Design review of the part shown in the three views and the two pictorial views. Dimensions are in mm from the part's minimum x, y and z. Round coordinates to 2 decimals unless told otherwise and drop trailing zeros. Write each loop counter-clockwise with the first axis right and the second up, starting at its lowest first coordinate (ties: lowest second). Pieces come first, ordered by that corner, then holes. Notation, with made-up numbers: (-1, -15.5) - (35, -15.5) arc R10 ccw to (35, 1.5) - close; hole circle Ø7 at (-36.5, 19.5). An arc over 180 degrees is marked (long way). One line per item, written item: value. Start each with the question number.
Q1. Add section C-C on x = 1.5. Write out the cut boundary in (y, z), and give its area (3 significant figures).
Q2. Add section B-B on z = 0.75. Write out the cut boundary in (x, y), and give its area (3 significant figures).
Q3. Clearance check with flat-ended pins moving along their axes: pin 1 Ø3 at (x, y) = (5, 40) entering from +Z; pin 2 Ø1.5 at (x, z) = (1, 3) entering from -Y. State where each tip first meets the part, or that it passes through.
Q4. For probe 1 along Y at (x, z) = (5.5, 2.9); probe 2 along Y at (x, z) = (3.25, 4.2); probe 3 along X at (y, z) = (4, 3.8), list the stretches that pass through material, from the lowest coordinate up.
Q5. Add section A-A on x = 5. Write out the cut boundary in (y, z), and give its area (3 significant figures).
Q6. Mouldability with a two-part tool opening along Y and no side actions: class the marked faces 1, 2 and 3 as +Y half, -Y half, draft (parallel to the pull), parting line (faces both ways), or undercut.
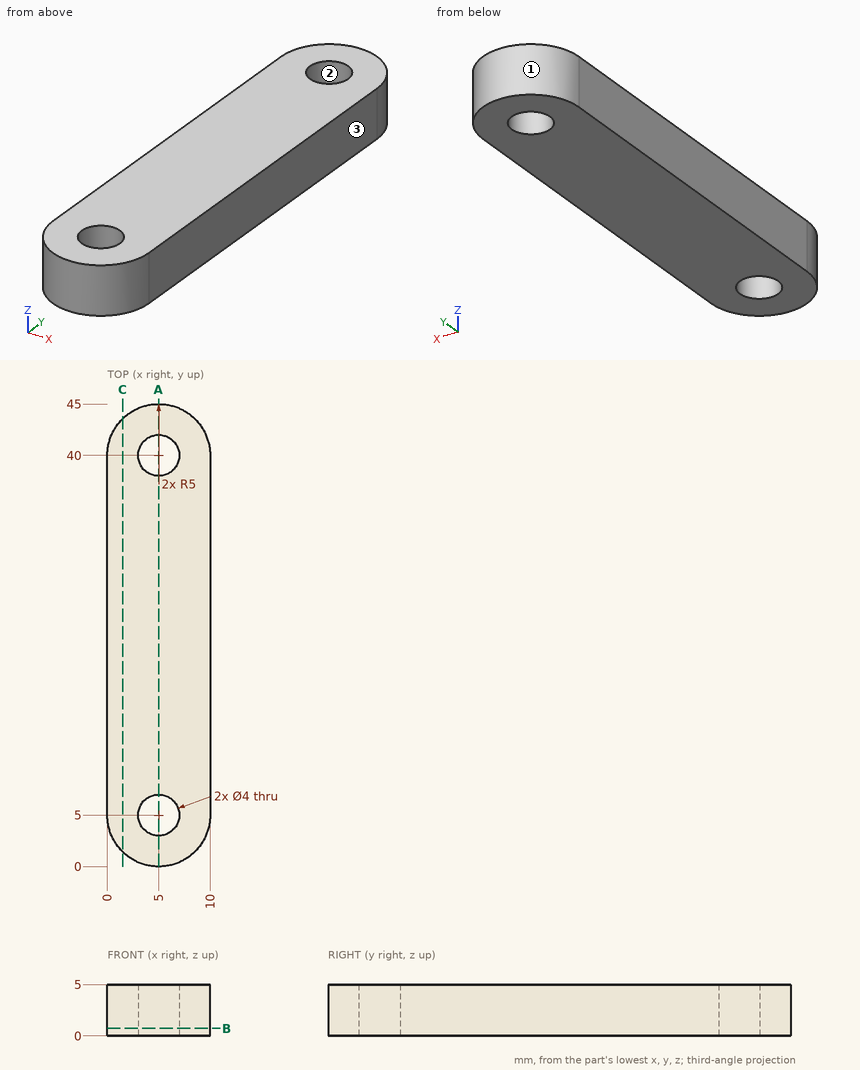
Result set:
1. outline: (1.43, 0) - (43.57, 0) - (43.57, 5) - (1.43, 5) - close
1. area: 211 mm^2
2. outline: (0, 5) arc R5 ccw to (10, 5) - (10, 40) arc R5 ccw to (0, 40) - close; hole circle Ø4 at (5, 5); hole circle Ø4 at (5, 40)
2. area: 403 mm^2
3. pin 1: passes through
3. pin 2: stops at y = 1.2
4. probe 1: y = 0.03 to 3.06, 6.94 to 38.06, 41.94 to 44.97
4. probe 2: y = 0.32 to 4.03, 5.97 to 39.03, 40.97 to 44.68
4. probe 3: x = 0.1 to 3.27, 6.73 to 9.9
5. outline: (0, 0) - (3, 0) - (3, 5) - (0, 5) - close; (7, 0) - (38, 0) - (38, 5) - (7, 5) - close; (42, 0) - (45, 0) - (45, 5) - (42, 5) - close
5. area: 185 mm^2
6. face 1: +Y half
6. face 2: undercut
6. face 3: draft
